Part print with two shaded views. Sizes in mm from the minimum x, y, z corner. Round coordinates to 2 decimals unless told otherwise and drop trailing zeros. Write each loop counter-clockwise with the first axis right and the second up, starting at its lowest first coordinate (ties: lowest second). Pieces come first, ordered by that corner, then holes. Notation, with made-up numbers: M 76.25,-33 L 84.25,-33 A9 ccw 84.25,-29 Z; hole C 67.25,-6 d8. An arc over 180 degrees is marked long. Use one line per item in the form item = value. Start each with the question number.
Item 1: Probe L1, parallel to Y at x = 17, z = 0.1 (1 decimal); L2, parallel to X at y = 8.5, z = 0.5 (1 decimal); L3, parallel to Y at x = 17.5, z = 0.4 (1 decimal). List the from-to ranges inside material, lowest first.
Item 2: Cut at C-C, the plane x = 22.5. Give the cut face in (y, z) (1 decimal), then the cut area to 3 significant figures.
Item 3: Cut at A-A, the plane y = 4.5. Give the cut face in (x, z).
Item 4: Cut at B-B, the plane z = 0.4. Give the cut face in (x, y) (1 decimal), then the cut area to 3 significant figures.
Item 5: Cut at D-D, the plane y = 6.5. Give the cut face in (x, z) (1 decimal).
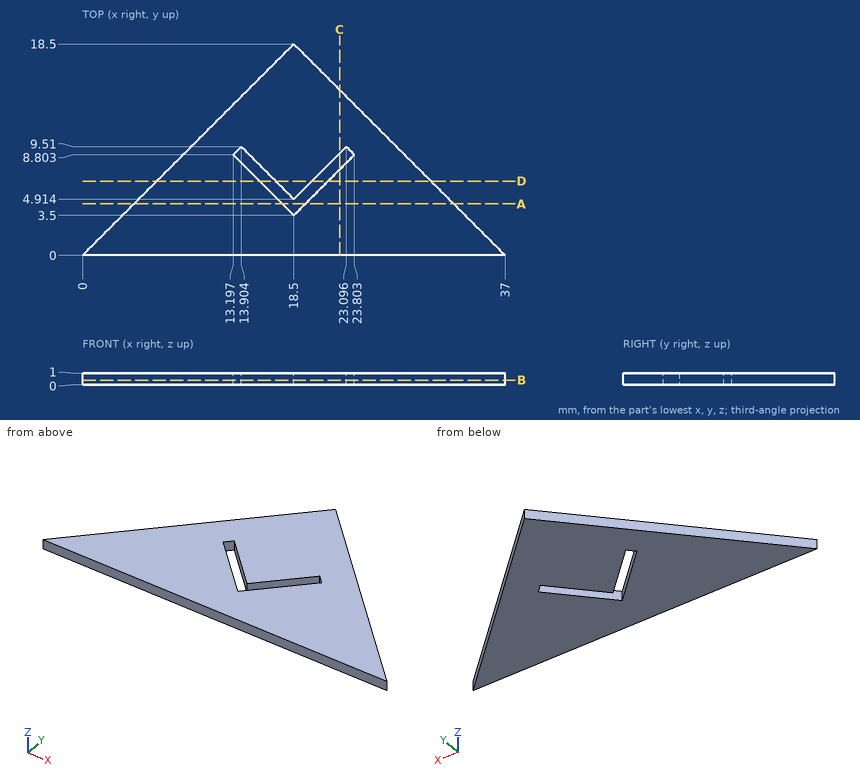
Model answer:
q1.L1 = 0 to 5, 6.4 to 17
q1.L2 = 8.5 to 13.5, 14.9 to 22.1, 23.5 to 28.5
q1.L3 = 0 to 4.5, 5.9 to 17.5
q2.outline = M 0,0 L 7.5,0 L 7.5,1 L 0,1 Z; M 8.9,0 L 14.5,0 L 14.5,1 L 8.9,1 Z
q2.area = 13.1 mm²
q3.outline = M 4.5,0 L 17.5,0 L 17.5,1 L 4.5,1 Z; M 19.5,0 L 32.5,0 L 32.5,1 L 19.5,1 Z
q4.outline = M 0,0 L 37,0 L 18.5,18.5 Z; hole M 13.2,8.8 L 18.5,3.5 L 23.8,8.8 L 23.1,9.5 L 18.5,4.9 L 13.9,9.5 Z
q4.area = 328 mm²
q5.outline = M 6.5,0 L 15.5,0 L 15.5,1 L 6.5,1 Z; M 16.9,0 L 20.1,0 L 20.1,1 L 16.9,1 Z; M 21.5,0 L 30.5,0 L 30.5,1 L 21.5,1 Z
